Geometry check sheet. Reference: the model listing, model coordinates, mm. A direction names the side the tool comes from. Give positions to 0.01 mm unless a question says otherwise; leave off trailing zeros. Write each loop counter-clockwise with the first axis right and the second up, starting at its lowest first coordinate (ties: lowest second). Pieces come first, ordered by that corner, then holes. Notation, with made-up numbers: M -14.75,11 L -0.75,11 A15 cw -0.75,38 Z; hole C 0.25,-12.75 d10. An arc over 180 degrees is marked long. Write each question's results on one line, items separated by ' | '.
```python
from build123d import *

# Parameters (mm, degrees)
PAD_DEPTH           = 235
SKETCH001_R         = 6
PAD001_DEPTH        = 40
SKETCH002_R         = 10
PAD002_DEPTH        = 20
LINEARPATTERN_COUNT = 3
LINEARPATTERN_PITCH = 65


with BuildPart() as part:
    # Sketch → Pad (new body)
    with BuildSketch(Plane.XZ):
        Polygon((0, 23.625182), (2.8, 23.625182), (2.8, 13.250815), (13.250815, 2.8), (80, 2.8), (80, 0), (0, 0), align=None)
    extrude(amount=PAD_DEPTH)

    # Sketch001 (on DatumPlane) → Pad001 (join)
    with BuildSketch(Plane(origin=(16, 0, 0), x_dir=(0, 1, 0), z_dir=(0.707107, 0, 0.707107))):
        with Locations((-50, 11.06395)):
            Circle(SKETCH001_R)
    pad001 = extrude(amount=PAD001_DEPTH)

    # Sketch002 (on DatumPlane) → Pad002 (join)
    with BuildSketch(Plane(origin=(16, 0, 0), x_dir=(0, 1, 0), z_dir=(0.707107, 0, 0.707107))):
        with Locations((-50, 11.382573)):
            Circle(SKETCH002_R)
    pad002 = extrude(amount=PAD002_DEPTH)

    # LinearPattern: Pad001, Pad002 ×3
    with Locations(*[(0, -i * LINEARPATTERN_PITCH, 0) for i in range(1, LINEARPATTERN_COUNT)]):
        add(pad001)
        add(pad002)


solid = part.part
```
Q1. Access from +Z, -Z, +X, -X, +Y, -Y to the whole of each face (thin tool, end or side, straight path). Record for faces 1 (the face through (28, 0, 1)), 2 (the face through (18.852, -45.696, 25.433)).
Answer key:
face 1: +Z, -Z, +X, -X, +Y | face 2: none
Q2. Section check C-C (x = 26.5). State how many separate pieces and enclosed holes the cut face has, then the cut area to 3 significant figures.
Answer key:
separate pieces: 4 | enclosed holes: 0 | area: 1,310 mm2
Q3. Section check B-B (x = 62). Enter the section's corners in (y, z), then the cut area to 3 significant figures.
Answer key:
outline: M -235,0 L 0,0 L 0,2.8 L -235,2.8 Z | area: 658 mm2
Q4. Depth check by flat-ended pin: P1, Ø0.8, axis at x = 1.5, y = -152, coming from the +Z side; P2, Ø6, axis at x = 10.5, y = -121, coming from the +Z side; P3, Ø1, axis at y = -148.5, z = 8, coming from the -X side; P4, Ø11.5, axis at y = -135.5, z = 20, coming from the +X side. Enter the tip coordinate at first touch or a pass-through.
Answer key:
P1: stops at z = 23.63 | P2: stops at z = 25.84 | P3: stops at x = 0 | P4: stops at x = 2.8
Q5. Section check D-D (y = -116.5). Enter the section's corners in (x, z), then the cut area to 3 significant figures.
Answer key:
outline: M 0,0 L 80,0 L 80,2.8 L 16.68,2.8 L 29.08,15.2 L 26.43,17.86 L 40.57,32 L 32.35,40.22 L 18.21,26.07 L 15.1,29.18 L 2.8,16.88 L 2.8,23.63 L 0,23.63 Z | area: 958 mm2
Q6. Section check A-A (y = -162.5). Enter the section's corners in (x, z).
Answer key:
outline: M 0,0 L 80,0 L 80,2.8 L 13.25,2.8 L 2.8,13.25 L 2.8,23.63 L 0,23.63 Z
Q7. Material ranges on probe 1 along Y at (x, z) = (15, 23.5); probe 2 along Y at (x, z) = (10, 20); probe 3 along Z at (x, y) = (67, -193), recorded low to high. Write a range as [from, to].
Answer key:
probe 1: y = [-188.04, -171.96], [-123.04, -106.96], [-58.04, -41.96] | probe 2: y = [-187.14, -172.86], [-122.14, -107.86], [-57.14, -42.86] | probe 3: z = [0, 2.8]
Q8. Release check for a two-part mould opening along Y. For faces 3 (the face through (15, -60, 15)), 4 (the face through (36.4, -180.08, 36.17)), 5 (the face through (28, -235, 1)) record: released by +Y, released by -Y, zero draft, split by the parting line, or undercut.
Answer key:
face 3: undercut | face 4: zero draft | face 5: released by -Y
